Source: CAD feature listing. Evaluate the final solid. Frame: model axes, mm. A direction names the side the tool comes from. Round coordinates to 2 decimals unless told otherwise and drop trailing zeros. Order: outer loops, then holes, each group sorted by start corner. A loop starts at its lowest first (then second) coordinate and runs counter-clockwise, first axis right, second up. Notation, with made-up numbers: (-9, 33) -> (31, 33) arc R28 cw to (31, 60) -> close; hole circle Ø6 at (33.25, 51.5). An arc over 180 degrees is marked (long way). Write item = value, one per line. Start each with the question number.
(1) Reachability of faces 1 (the face through (-40.393, -35.533, 1.479)), 2 (the face through (0, -48, 10)) from +Z, -Z, +X, -X, +Y, -Y: full face, straight path, thin tool, end or side. Return the list, or none.
(2) Cut plane D-D on y = -32.8. Return the cut outline in (x, z), then the cut area to 3 significant figures.
(3) Cut plane A-A on x = -41. Return the cut outline in (y, z).
(4) Cut plane C-C on y = 32.8. Return the cut outline in (x, z).
(5) Cut plane B-B on y = 9. Return the cut outline in (x, z).
(6) Ray query, line 1 (Y direction, x = -41, z = 1.7); line 2 (Z direction, x = -13.5, y = 37); line 3 (Y direction, x = 74.5, z = 2.75). Return the intervals inside material, ascending.
(7) Contact query for flat-ended pins moving along their axis: pin 1 Ø2.5 at (x, z) = (-62.5, 1.5) entering from -Y; pin 2 Ø1.5 at (x, y) = (-34, 30.5) entering from +Z. Output: stop coordinate, or through.
(8) Draft query along X for faces 3 (the face through (-40.635, 35.576, 1.479)), 4 (the face through (-1, 1, 3)). Return one class per face: released by +X, released by -X, zero draft, split by the parting line, or undercut.
from build123d import *

# Parameters (mm, degrees)
SKETCH2_W           = 175
SKETCH2_H           = 96
BOSS_EXTRUDE1_DEPTH = 3
SKETCH3_W           = 12
SKETCH3_H           = 12
SKETCH3_W_2         = 13
SKETCH3_H_2         = 10.5
SKETCH3_W_3         = 27
SKETCH3_H_3         = 14
CUT_EXTRUDE1_DEPTH  = 10
SKETCH4_W           = 14
SKETCH4_H           = 26
CUT_EXTRUDE2_DEPTH  = 10
SKETCH5_W           = 12
SKETCH5_H           = 12
SKETCH5_W_2         = 6
SKETCH5_H_2         = 6
CUT_EXTRUDE3_DEPTH  = 10
SKETCH7_R           = 2.8
CUT_EXTRUDE4_DEPTH  = 10
SKETCH9_W           = 25
SKETCH9_H           = 15.829859375
BOSS_EXTRUDE2_DEPTH = 3
SKETCH10_W          = 27
SKETCH10_H          = 14
CUT_EXTRUDE5_DEPTH  = 10
SKETCH11_W          = 14
SKETCH11_H          = 14
CUT_EXTRUDE6_DEPTH  = 10
SKETCH12_W          = 14
SKETCH12_H          = 14
CUT_EXTRUDE7_DEPTH  = 10
SKETCH13_W          = 14
SKETCH13_H          = 14
CUT_EXTRUDE8_DEPTH  = 10


with BuildPart() as part:
    # Sketch2 → Boss-Extrude1 (new body)
    with BuildSketch(Plane.XY):
        Rectangle(SKETCH2_W, SKETCH2_H)
    extrude(amount=BOSS_EXTRUDE1_DEPTH)

    # Sketch3 → Cut-Extrude1 (cut)
    with BuildSketch(Plane(origin=(0, 0, 0), x_dir=(-1, 0, 0), z_dir=(0, 0, -1))):
        with Locations((53.5, 34)):
            Rectangle(SKETCH3_W, SKETCH3_H)
        with Locations((69.5, 34.75)):
            Rectangle(SKETCH3_W_2, SKETCH3_H_2)
        with Locations((-42, 34)):
            Rectangle(SKETCH3_W_3, SKETCH3_H_3)
        with Locations((-48.5, 34)):
            Rectangle(SKETCH3_W, SKETCH3_H, mode=Mode.SUBTRACT)
        with Locations((-35.5, 34)):
            Rectangle(SKETCH3_W, SKETCH3_H, mode=Mode.SUBTRACT)
    extrude(amount=-CUT_EXTRUDE1_DEPTH, mode=Mode.SUBTRACT)

    # Sketch4 → Cut-Extrude2 (cut)
    with BuildSketch(Plane(origin=(0, 0, 0), x_dir=(-1, 0, 0), z_dir=(0, 0, -1))):
        with Locations((-42.5, 0)):
            Rectangle(SKETCH4_W, SKETCH4_H)
    extrude(amount=-CUT_EXTRUDE2_DEPTH, mode=Mode.SUBTRACT)

    # Sketch5 → Cut-Extrude3 (cut)
    with BuildSketch(Plane(origin=(0, 0, 0), x_dir=(-1, 0, 0), z_dir=(0, 0, -1))):
        with Locations((-42, -33)):
            Rectangle(SKETCH5_W, SKETCH5_H)
        with Locations((53.5, -33)):
            Rectangle(SKETCH5_W, SKETCH5_H)
        with Locations((78.5, -33)):
            Rectangle(SKETCH5_W_2, SKETCH5_H_2)
    extrude(amount=-CUT_EXTRUDE3_DEPTH, mode=Mode.SUBTRACT)

    # Sketch7 → Cut-Extrude4 (cut)
    with BuildSketch(Plane(origin=(0, 0, 0), x_dir=(-1, 0, 0), z_dir=(0, 0, -1))):
        with Locations((41, 32.8)):
            Circle(SKETCH7_R)
        with Locations((41, -32.8)):
            Circle(SKETCH7_R)
    extrude(amount=-CUT_EXTRUDE4_DEPTH, mode=Mode.SUBTRACT)

    # Sketch9 → Boss-Extrude2 (add)
    with BuildSketch(Plane.XZ.offset(48)):
        with Locations((0, 7.914929688)):
            Rectangle(SKETCH9_W, SKETCH9_H)
    extrude(amount=BOSS_EXTRUDE2_DEPTH)

    # Sketch10 → Cut-Extrude5 (cut)
    with BuildSketch(Plane(origin=(0, 0, 0), x_dir=(-1, 0, 0), z_dir=(0, 0, -1))):
        with Locations((-42, 34)):
            Rectangle(SKETCH10_W, SKETCH10_H)
    extrude(amount=-CUT_EXTRUDE5_DEPTH, mode=Mode.SUBTRACT)

    # Sketch11 → Cut-Extrude6 (cut)
    with BuildSketch(Plane(origin=(0, 0, 0), x_dir=(-1, 0, 0), z_dir=(0, 0, -1))):
        with Locations((53.5, 34)):
            Rectangle(SKETCH11_W, SKETCH11_H)
    extrude(amount=-CUT_EXTRUDE6_DEPTH, mode=Mode.SUBTRACT)

    # Sketch12 → Cut-Extrude7 (cut)
    with BuildSketch(Plane(origin=(0, 0, 0), x_dir=(-1, 0, 0), z_dir=(0, 0, -1))):
        with Locations((53.5, -33)):
            Rectangle(SKETCH12_W, SKETCH12_H)
    extrude(amount=-CUT_EXTRUDE7_DEPTH, mode=Mode.SUBTRACT)

    # Sketch13 → Cut-Extrude8 (cut)
    with BuildSketch(Plane(origin=(0, 0, 0), x_dir=(-1, 0, 0), z_dir=(0, 0, -1))):
        with Locations((-42, -33)):
            Rectangle(SKETCH13_W, SKETCH13_H)
    extrude(amount=-CUT_EXTRUDE8_DEPTH, mode=Mode.SUBTRACT)


solid = part.part
Evaluation:
q1.face_1 = +Z, -Z
q1.face_2 = +Z, +X, -X, +Y
q2.outline = (-87.5, 0) -> (-81.5, 0) -> (-81.5, 3) -> (-87.5, 3) -> close; (-75.5, 0) -> (-60.5, 0) -> (-60.5, 3) -> (-75.5, 3) -> close; (-46.5, 0) -> (-43.8, 0) -> (-43.8, 3) -> (-46.5, 3) -> close; (-38.2, 0) -> (35, 0) -> (35, 3) -> (-38.2, 3) -> close; (49, 0) -> (87.5, 0) -> (87.5, 3) -> (49, 3) -> close
q2.area = 406 mm^2
q3.outline = (-48, 0) -> (-35.6, 0) -> (-35.6, 3) -> (-48, 3) -> close; (-30, 0) -> (30, 0) -> (30, 3) -> (-30, 3) -> close; (35.6, 0) -> (48, 0) -> (48, 3) -> (35.6, 3) -> close
q4.outline = (-87.5, 0) -> (-76, 0) -> (-76, 3) -> (-87.5, 3) -> close; (-63, 0) -> (-60.5, 0) -> (-60.5, 3) -> (-63, 3) -> close; (-46.5, 0) -> (-43.8, 0) -> (-43.8, 3) -> (-46.5, 3) -> close; (-38.2, 0) -> (28.5, 0) -> (28.5, 3) -> (-38.2, 3) -> close; (55.5, 0) -> (87.5, 0) -> (87.5, 3) -> (55.5, 3) -> close
q5.outline = (-87.5, 0) -> (35.5, 0) -> (35.5, 3) -> (-87.5, 3) -> close; (49.5, 0) -> (87.5, 0) -> (87.5, 3) -> (49.5, 3) -> close
q6.line_1 = -48 to -35.6, -30 to 30, 35.6 to 48
q6.line_2 = 0 to 3
q6.line_3 = -48 to 48
q7.pin_1 = -48
q7.pin_2 = 3
q8.face_3 = undercut
q8.face_4 = zero draft
